Read the model definition and answer for the solid it produces. Units are mm, in the model's axes. Face numbers are marked on the shaded views. A direction names the side the tool comes from. Coordinates: 2 decimals unless noted, no trailing zeros. Order: outer loops, then holes, each group sorted by start corner. A loop starts at its lowest first (then second) coordinate and runs counter-clockwise, first axis right, second up. Notation, with made-up numbers: (20.5, 11) -> (77.5, 11) arc R21 cw to (77.5, 29) -> close; hole circle Ø8 at (37.25, -21). An arc over 180 degrees is marked (long way). Answer in a Markdown table with one row per item.
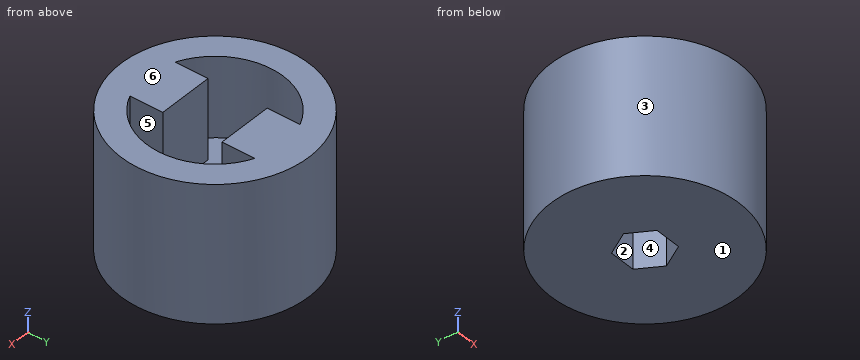
from build123d import *

# Parameters (mm, degrees)
SKETCH1_R           = 8.25
BOSS_EXTRUDE1_DEPTH = 12
CUT_EXTRUDE1_DEPTH  = 7
CUT_EXTRUDE2_DEPTH  = 17.736935203


with BuildPart() as part:
    # Sketch1 → Boss-Extrude1 (new body)
    with BuildSketch(Plane.XY):
        Circle(SKETCH1_R)
    extrude(amount=BOSS_EXTRUDE1_DEPTH)

    # Sketch2 → Cut-Extrude1 (cut)
    with BuildSketch(Plane.XY.offset(12)):
        with BuildLine():
            Line((-2.425, 2.6), (-2.425, 5.488112153))
            ThreePointArc((-2.425, 5.488112153), (-6, 0), (-2.425, -5.488112153))
            Line((-2.425, -5.488112153), (-2.425, -2.6))
            Line((-2.425, -2.6), (2.425, -2.6))
            Line((2.425, -2.6), (2.425, -5.488112153))
            ThreePointArc((2.425, -5.488112153), (5.027424788, -3.274904579), (6, 0))
            ThreePointArc((6, 0), (5.027424788, 3.274904579), (2.425, 5.488112153))
            Line((2.425, 5.488112153), (2.425, 2.6))
            Line((2.425, 2.6), (-2.425, 2.6))
        make_face()
    extrude(amount=-CUT_EXTRUDE1_DEPTH, mode=Mode.SUBTRACT)

    # Sketch3 → Cut-Extrude2 (cut, through all)
    with BuildSketch(Plane(origin=(0, 0, 0), x_dir=(-1, 0, 0), z_dir=(0, 0, -1))):
        Polygon((2.309401077, 0), (1.154700538, 2), (-1.154700538, 2), (-2.309401077, 0), (-1.154700538, -2), (1.154700538, -2), align=None)
    extrude(amount=-CUT_EXTRUDE2_DEPTH, mode=Mode.SUBTRACT)


solid = part.part
Q1. For a pull along X with two mould halves and no side action, classify the marked faces 1, 2 and 3 as pulls with the +X half, pulls with the -X half, needs draft (parallel to the pull), parting line crosses it, or undercut.
Outcome:
| item | result |
|---|---|
| face 1 | needs draft |
| face 2 | undercut |
| face 3 | parting line crosses it |
Q2. The part is cut by section C-C (y = -0.25). Write down the section's boundary in (x, z), then the cut area to 3 significant figures.
Outcome:
| item | result |
|---|---|
| outline | (-8.25, 0) -> (-2.17, 0) -> (-2.17, 5) -> (-5.99, 5) -> (-5.99, 12) -> (-8.25, 12) -> close; (2.17, 0) -> (8.25, 0) -> (8.25, 12) -> (5.99, 12) -> (5.99, 5) -> (2.17, 5) -> close |
| area | 92.3 mm² |
Q3. For the marked faces 4, 5 and 6, determine the directions among +Z, -Z, +X, -X, +Y, -Y from which every point of the face is accessible in a straight line to the end or side of a thin tool.
Outcome:
| item | result |
|---|---|
| face 4 | +Z, -Z |
| face 5 | +Z |
| face 6 | +Z, +X, -X, +Y, -Y |
Q4. The part is cut by section D-D (z = 1.75). Write down the section's boundary in (x, y), then the cut area to 3 significant figures.
Outcome:
| item | result |
|---|---|
| outline | circle Ø16.5 at (0, 0); hole (-2.31, 0) -> (-1.15, -2) -> (1.15, -2) -> (2.31, 0) -> (1.15, 2) -> (-1.15, 2) -> close |
| area | 200 mm² |
Q5. Given pin 1 (4 mm diameter, centred on x = -6, z = 8, fed in from -Y); pin 2 (1.5 mm diameter, centred on x = -4, y = -1, fed in from +Z); pin 3 (2 mm diameter, centred on y = -4, z = 10, fed in from -X); pin 4 (4 mm diameter, centred on x = -3.5, y = -4, fed in from -Z), each flat-ended and moving along its own axis, determine where each tip first touches the part or whether it passes through.
Outcome:
| item | result |
|---|---|
| pin 1 | y = -7.22 |
| pin 2 | z = 5 |
| pin 3 | x = -7.69 |
| pin 4 | z = 0 |
Q6. The part is cut by section B-B (x = -1.5). Write down the section's boundary in (y, z).
Outcome:
| item | result |
|---|---|
| outline | (-8.11, 0) -> (-1.4, 0) -> (-1.4, 5) -> (-2.6, 5) -> (-2.6, 12) -> (-8.11, 12) -> close; (1.4, 0) -> (8.11, 0) -> (8.11, 12) -> (2.6, 12) -> (2.6, 5) -> (1.4, 5) -> close |
Q7. The part is cut by section A-A (z = 6.5). Write down the section's boundary in (x, y) (3 decimals).
Outcome:
| item | result |
|---|---|
| outline | circle Ø16.5 at (0, 0); hole (-2.425, -5.488) -> (-2.425, -2.6) -> (2.425, -2.6) -> (2.425, -5.488) arc R6 ccw to (2.425, 5.488) -> (2.425, 2.6) -> (-2.425, 2.6) -> (-2.425, 5.488) arc R6 ccw to start |
Q8. Consider line 1 (X direction, y = -3, z = 10.5) (3 decimals); line 2 (X direction, y = 4, z = 8) (3 decimals); line 3 (X direction, y = -0.25, z = 5.5). Determine where each line is inside the solid, lowest interval first.
Outcome:
| item | result |
|---|---|
| line 1 | -7.685 to -5.196, -2.425 to 2.425, 5.196 to 7.685 |
| line 2 | -7.215 to -4.472, -2.425 to 2.425, 4.472 to 7.215 |
| line 3 | -8.25 to -5.99, 5.99 to 8.25 |
